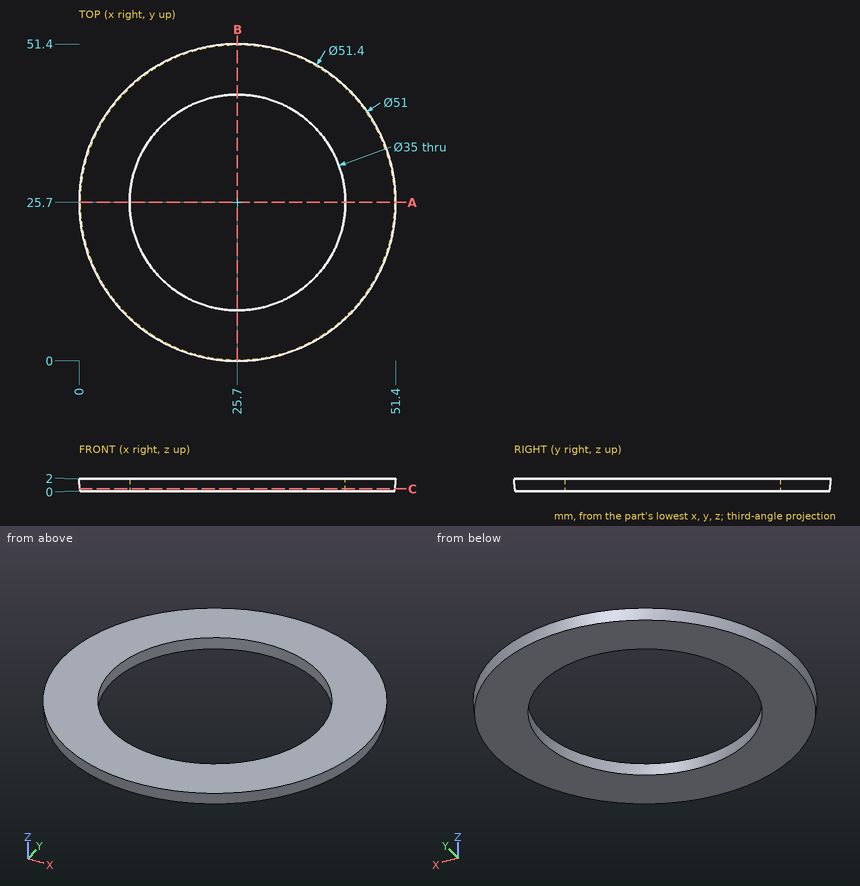
Input: dimensioned drawing with shaded views. Units: mm. Origin: part minimum x, y, z. Give positions to 0.01 mm unless a question says otherwise; leave off trailing zeros. Write each loop counter-clockwise with the first axis right and the second up, starting at its lowest first coordinate (ties: lowest second). Pieces come first, ordered by that corner, then holes. Notation, with made-up numbers: M 6,82 L 58,82 A13 ccw 58,99 Z; hole C 36.5,3 d5. An arc over 180 degrees is marked long. Return JSON: item names as keys, results as strings. Group by question number.
1) Cut plane A-A, the plane y = 25.7. Output: boundary loops of the cut face in (x, z).
2) Cut plane C-C, the plane z = 0.4. Output: boundary loops of the cut face in (x, y), plus the area to 3 significant figures.
3) Pin query (flat end, axial travel): P1, Ø1, axis at x = 32.5, y = 10.5, coming from the -Z side. Return the tip coordinate at first contact, or that it passes through.
4) Material intervals for line 1 along Y through (x, z) = (29.5, 1.4); line 2 along Y through (x, z) = (25.7, 0.4); line 3 along X through (y, z) = (20, 1.2), sorted ascending. Write a range as [from, to].
Recorded:
{
 "1": {"outline": "M 0,2 L 0.2,0 L 8.2,0 L 8.2,2 Z; M 43.2,0 L 51.2,0 L 51.4,2 L 43.2,2 Z"},
 "2": {"outline": "C 25.7,25.7 d51.08; hole C 25.7,25.7 d35", "area": "1,090 mm²"},
 "3": {"P1": "passes through"},
 "4": {"line 1": "y = [0.34, 8.62], [42.78, 51.06]", "line 2": "y = [0.16, 8.2], [43.2, 51.24]", "line 3": "x = [0.72, 9.15], [42.25, 50.68]"}
}
